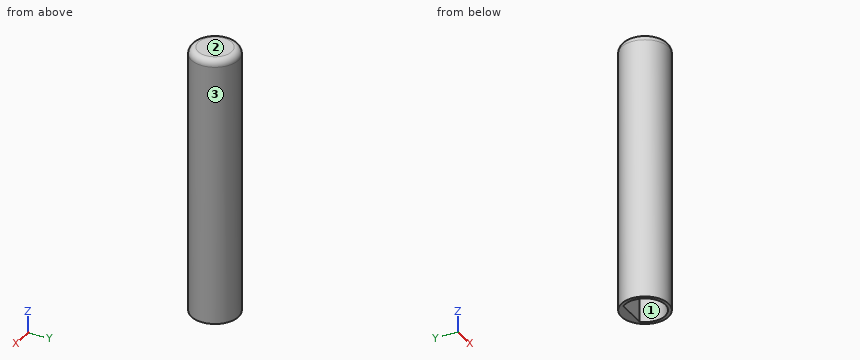
from build123d import *

# Parameters (mm, degrees)
ESBO_O2_R                = 1.75
RESSALTO_EXTRUS_O1_DEPTH = 9.3
ESBO_O3_R                = 1.75
RESSALTO_EXTRUS_O2_DEPTH = 10.7
FILETE1_R                = 0.5


with BuildPart() as part:
    # Esboço2 → Ressalto-extrusão1 (new body)
    with BuildSketch(Plane.XY):
        with Locations((0, 0.25)):
            Circle(ESBO_O2_R)
        with BuildLine():
            Line((1.118033989, 1.25), (-1.118033989, 1.25))
            ThreePointArc((-1.118033989, 1.25), (0, -1.25), (1.118033989, 1.25))
        make_face(mode=Mode.SUBTRACT)
    extrude(amount=RESSALTO_EXTRUS_O1_DEPTH)

    # Esboço3 → Ressalto-extrusão2 (add)
    with BuildSketch(Plane.XY.offset(9.3)):
        with Locations((0, 0.25)):
            Circle(ESBO_O3_R)
    extrude(amount=RESSALTO_EXTRUS_O2_DEPTH)

    # Filete1
    filete1_edges = [part.edges().sort_by_distance(p)[0] for p in [
        (-1.75, 0.25, 20),
    ]]
    fillet(filete1_edges, radius=FILETE1_R)


solid = part.part
The listing builds one solid part. Answer for the finished solid, in the listing's coordinates (mm). Face numbers are marked on the shaded views. Give positions to 0.01 mm unless a question says otherwise; leave off trailing zeros. Loops run counter-clockwise (first coordinate to the right, second up) from the corner with the lowest first, then second, coordinate; pieces in that order, holes last. Notation, with made-up numbers: (25.5, 83.25) - (73.5, 83.25) arc R27 ccw to (73.5, 106.25) - close; hole circle Ø9 at (-39, 30). An arc over 180 degrees is marked (long way). Use one line per item in the form item = value.
1. Section B-B on x = 0 is taken. Give the vertices of the cut face in (y, z).
Calculated:
outline = (-1.5, 0) - (-1.25, 0) - (-1.25, 9.3) - (1.25, 9.3) - (1.25, 0) - (2, 0) - (2, 19.5) arc R0.5 ccw to (1.5, 20) - (-1, 20) arc R0.5 ccw to (-1.5, 19.5) - close
2. The mould has two halves that part along X. Classify the marked faces 1, 2 and 3: pulls with the +X half, pulls with the -X half, needs draft (parallel to the pull), parting line crosses it, or undercut.
Calculated:
face_1 = undercut
face_2 = needs draft
face_3 = parting line crosses it
3. Find the intervals of material crossed by line 1 along Y through (x, z) = (0, 4.75); line 2 along X through (y, z) = (-0.55, 3.75); line 3 along Z through (x, y) = (0.45, 0.7), in increasing order. Write a range as [from, to].
Calculated:
line_1 = [-1.5, -1.25], [1.25, 2]
line_2 = [-1.56, -1.27], [1.27, 1.56]
line_3 = [9.3, 20]
4. Section A-A on y = 0.25 is taken. Give the vertices of the cut face in (x, z).
Calculated:
outline = (-1.75, 0) - (-1.5, 0) - (-1.5, 9.3) - (1.5, 9.3) - (1.5, 0) - (1.75, 0) - (1.75, 19.5) arc R0.5 ccw to (1.25, 20) - (-1.25, 20) arc R0.5 ccw to (-1.75, 19.5) - close
5. Section C-C on z = 5.5 is taken. Give the vertices of the cut face in (x, y).
Calculated:
outline = circle Ø3.5 at (0, 0.25); hole (-1.12, 1.25) arc R1.5 ccw (long way) to (1.12, 1.25) - close
